Study the drawing (mm; zero at the part's minimum x, y, z) and answer. Give positions to 0.01 mm unless a question says otherwise; leave off trailing zeros. Order: outer loops, then holes, each group sorted by start corner. A loop starts at its lowest first (then second) coordinate and runs counter-clockwise, first axis right, second up.
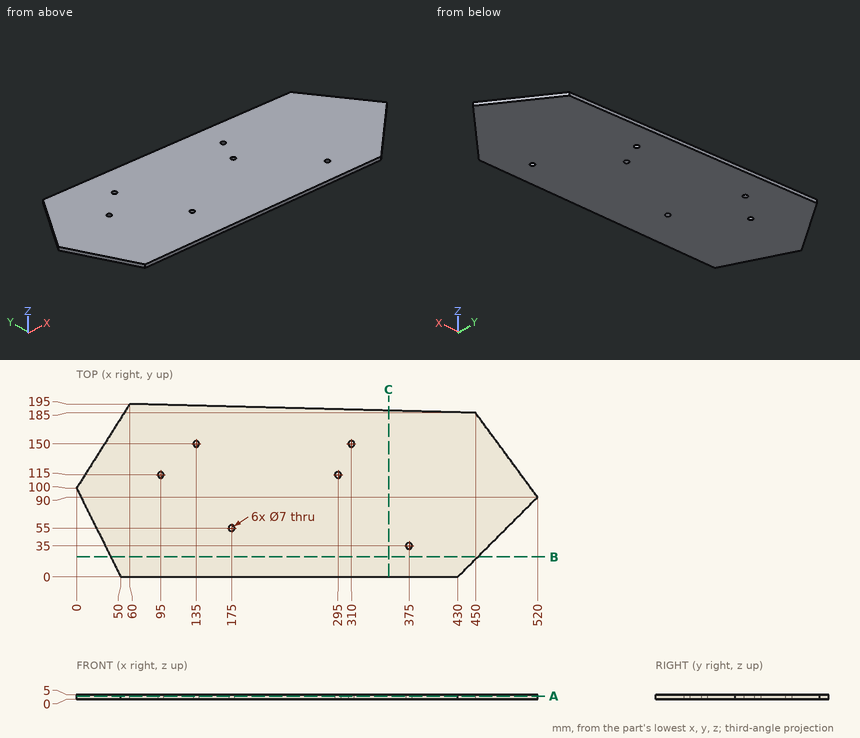
1) Straight lines are drawn through the part: probe 1 along X at (y, z) = (118, 4.75); probe 2 along Y at (x, z) = (175, 3.6); probe 3 along Y at (x, z) = (375, 1). For each, find the intervals that lie inside material, in ascending order.
Geometry says:
probe 1: x = 11.37 to 93.2, 96.8 to 293.2, 296.8 to 499.37
probe 2: y = 0 to 51.5, 58.5 to 192.05
probe 3: y = 0 to 31.5, 38.5 to 186.92
2) Find section A-A (z = 3.7). Write down the section's boundary in (x, y), then the cut area to 3 significant figures.
Geometry says:
outline: (0, 100) - (50, 0) - (430, 0) - (520, 90) - (450, 185) - (60, 195) - close; hole circle Ø7 at (95, 115); hole circle Ø7 at (135, 150); hole circle Ø7 at (175, 55); hole circle Ø7 at (295, 115); hole circle Ø7 at (310, 150); hole circle Ø7 at (375, 35)
area: 85,800 mm2
3) Find section B-B (y = 22.5). Write down the section's boundary in (x, z).
Geometry says:
outline: (38.75, 0) - (452.5, 0) - (452.5, 5) - (38.75, 5) - close
4) Given P1, Ø6.5, axis at x = 95, y = 115, coming from the +Z side; P2, Ø1.5, axis at x = 410.5, z = 2.5, coming from the +Y side, each flat-ended and moving along its own axis, determine where each tip first touches the part or whether it passes through.
Geometry says:
P1: passes through
P2: stops at y = 186.03
5) Find section C-C (x = 352). Write down the section's boundary in (y, z).
Geometry says:
outline: (0, 0) - (187.51, 0) - (187.51, 5) - (0, 5) - close
